Check sheet for the modelled part. Datum: model origin and axes. Units: mm. A direction names the side the tool comes from. Give positions to 0.01 mm unless a question says otherwise; leave off trailing zeros. Order: outer loops, then holes, each group sorted by start corner. A loop starts at its lowest first (then second) coordinate and runs counter-clockwise, first axis right, second up.
```python
from build123d import *

# Parameters (mm, degrees)
SKETCH_1_R          = 3
EXTRUDE_1_DEPTH     = 1
SKETCH_2_R          = 1.5
EXTRUDE_2_DEPTH     = 8
FILLET_1_R          = 0.15
CHAMFER_1_SIZE      = 0.2
CUT_EXTRUDE_1_DEPTH = 0.5


with BuildPart() as part:
    # 草图1 → 凸台-拉伸1 (new body)
    with BuildSketch(Plane(origin=(0, 0, 0), x_dir=(1, 0, 0), z_dir=(0, 1, 0))):
        Circle(SKETCH_1_R)
    extrude(amount=EXTRUDE_1_DEPTH)

    # 草图2 → 凸台-拉伸2 (add)
    with BuildSketch(Plane.XZ):
        Circle(SKETCH_2_R)
    extrude(amount=EXTRUDE_2_DEPTH)

    # 圆角1
    fillet_1_edges = [part.edges().sort_by_distance(p)[0] for p in [
        (-3, 0, 0),
        (-3, 1, 0),
    ]]
    fillet(fillet_1_edges, radius=FILLET_1_R)

    # 倒角1
    chamfer_1_edges = [part.edges().sort_by_distance(p)[0] for p in [
        (-1.5, -8, 0),
    ]]
    chamfer(chamfer_1_edges, length=CHAMFER_1_SIZE)

    # 草图3 → 切除-拉伸1 (cut)
    with BuildSketch(Plane(origin=(0, 1, 0), x_dir=(1, 0, 0), z_dir=(0, 1, 0))):
        Polygon((1.154700538, 0), (0.577350269, 1), (-0.577350269, 1), (-1.154700538, 0), (-0.577350269, -1), (0.577350269, -1), align=None)
    extrude(amount=-CUT_EXTRUDE_1_DEPTH, mode=Mode.SUBTRACT)


solid = part.part
```
(1) Cross-section at B-B on y = -4. Enter the section's corners in (x, z), then the cut area to 3 significant figures.
Response values:
outline: circle Ø3 at (0, 0)
area: 7.07 mm2
(2) Release check for a two-part mould opening along Z. For faces 3 (the face through (0, -8, 0)), 4 (the face through (-1.5, -3.85, 0.07)), 5 (the face through (0, 0.5, 0)) record: released by +Z, released by -Z, zero draft, split by the parting line, or undercut.
Response values:
face 3: zero draft
face 4: split by the parting line
face 5: undercut
(3) Set-up check for faces 1 (the face through (1.2, 0, 1.2)), 2 (the face through (0, 1, 1.2)): record each of +Z, -Z, +X, -X, +Y, -Y from which the full face is reachable in a straight line by a thin tool's end or side.
Response values:
face 1: -Y
face 2: +Z, -Z, +X, -X, +Y
(4) Cross-section at A-A on x = 0. Enter the section's corners in (y, z), then the cut area to 3 significant figures.
Response values:
outline: (-8, -1.3) - (-7.8, -1.5) - (0, -1.5) - (0, -2.85) arc R0.15 ccw to (0.15, -3) - (0.85, -3) arc R0.15 ccw to (1, -2.85) - (1, -1) - (0.5, -1) - (0.5, 1) - (1, 1) - (1, 2.85) arc R0.15 ccw to (0.85, 3) - (0.15, 3) arc R0.15 ccw to (0, 2.85) - (0, 1.5) - (-7.8, 1.5) - (-8, 1.3) - close
area: 28.9 mm2
(5) Material ranges on L1, parallel to Y at x = -2.25, z = 0.25; L2, parallel to Y at x = -0.25, z = 0.25; L3, parallel to Z at x = -0.75, y = -0.25, recorded low to high.
Response values:
L1: y = 0 to 1
L2: y = -8 to 0.5
L3: z = -1.3 to 1.3
(6) Gauge pin test, flat ends, axial feed: pin 1 Ø0.6 at (x, y) = (-0.5, 1) entering from -Z; pin 2 Ø0.6 at (x, y) = (0.5, 0.5) entering from +Z; pin 3 Ø1.6 at (x, z) = (0, 0.5) entering from +Y; pin 4 Ø1 at (x, y) = (-1.5, -1) entering from +Z. Record the tip position at first contact, or that the pin passes through.
Response values:
pin 1: stops at z = -2.99
pin 2: stops at z = 2.99
pin 3: stops at y = 1
pin 4: stops at z = 1.12
